Autodesk Inventor part; units mm, degrees
ref_plane "YZ Plane" through (0, 0, 0) normal (1, 0, 0) x (0, 1, 0)
ref_plane "XZ Plane" through (0, 0, 0) normal (0, 1, 0) x (-1, 0, 0)
ref_plane "XY Plane" through (0, 0, 0) normal (0, 0, 1) x (1, 0, 0)
sketch "Sketch1" plane through (0, 0, 0) normal (0, 0, 1) x (1, 0, 0)
  line L0 (0, 0) -> (115, 0)
  line L1 (115, 0) -> (115, 105)
  line L2 (115, 105) -> (0, 105)
  line L3 (0, 105) -> (0, 0)
  circle A0 centre (57.5, 52.5) radius 4.5
  line L4 (27.5, 22.5) -> (87.5, 22.5) construction
  line L5 (87.5, 22.5) -> (87.5, 82.5) construction
  line L6 (87.5, 82.5) -> (27.5, 82.5) construction
  line L7 (27.5, 82.5) -> (27.5, 22.5) construction
  circle A1 centre (87.5, 82.5) radius 2.5
  circle A2 centre (27.5, 82.5) radius 2.5
  circle A3 centre (27.5, 22.5) radius 2.5
  circle A4 centre (87.5, 22.5) radius 2.5
  point P0 (57.5, 0)
  point P1 (0, 52.5)
  point P2 (27.5, 52.5)
  point P3 (57.5, 82.5)
  dimension "d0" = 115
  dimension "d1" = 105
  dimension "d2" = 9
  dimension "d3" = 60
  dimension "d4" = 60
  dimension "d5" = 5
  dimension "d6" = 5
  dimension "d7" = 5
  dimension "d8" = 5
extrude "Extrusion1" add sketch "Sketch1" along normal blind 20
fillet "Fillet1" radius 20 4 edges at (0, 105, 10) (115, 105, 10) (115, 0, 10) (0, 0, 10)
sketch "Sketch5" plane through (0, 0, 20) normal (0, 0, 1) x (1, 0, 0)
  circle A0 centre (27.5, 82.5) radius 2.5
  circle A1 centre (87.5, 82.5) radius 2.5
  circle A2 centre (87.5, 22.5) radius 2.5
  circle A3 centre (27.5, 22.5) radius 2.5
  circle A4 centre (87.5, 82.5) radius 6.5
  circle A5 centre (87.5, 22.5) radius 6.5
  circle A6 centre (27.5, 22.5) radius 6.5
  circle A7 centre (27.5, 82.5) radius 6.5
  point P0 (0, 0)
  dimension "d18" = 13
  dimension "d19" = 13
  dimension "d20" = 13
  dimension "d21" = 13
extrude "Extrusion4" cut sketch "Sketch5" against normal blind 5 contours A0 | A1 | A2 | A3 | A4 | A5 | A6 | A7
properties part number "AA030" material "ABS Plastic"
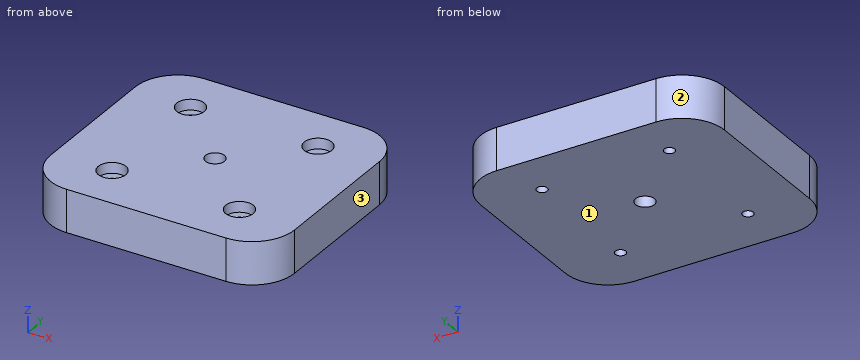
Check sheet for the modelled part. Datum: model origin and axes. Units: mm. Face numbers are marked on the shaded views. Give positions to 0.01 mm unless a question says otherwise; leave off trailing zeros. Write each loop counter-clockwise with the first axis right and the second up, starting at its lowest first coordinate (ties: lowest second). Pieces come first, ordered by that corner, then holes. Notation, with made-up numbers: (86, 1.25) -> (95, 1.25) arc R22 ccw to (95, 9.25) -> close; hole circle Ø1 at (-38, 55.25). An arc over 180 degrees is marked (long way). Write item = value, one per line.
Item 1: Sectioned sample at A-A on z = 17. Record the boundary of the cut face in (x, y).
Output:
outline = (0, 20) arc R20 ccw to (20, 0) -> (95, 0) arc R20 ccw to (115, 20) -> (115, 85) arc R20 ccw to (95, 105) -> (20, 105) arc R20 ccw to (0, 85) -> close; hole circle Ø13 at (27.5, 22.5); hole circle Ø13 at (27.5, 82.5); hole circle Ø9 at (57.5, 52.5); hole circle Ø13 at (87.5, 22.5); hole circle Ø13 at (87.5, 82.5)
Item 2: Scan lines: probe 1 along Y at (x, z) = (27.5, 5.75); probe 2 along X at (y, z) = (82.5, 10.75); probe 3 along Y at (x, z) = (24, 15.5). Record each from-to range of solid material in increasing order. Write a range as from..to.
Output:
probe_1 = 0..20, 25..80, 85..105
probe_2 = 0..25, 30..85, 90..115
probe_3 = 0..17.02, 27.98..77.02, 87.98..105
Item 3: Gauge pin test, flat ends, axial feed: pin 1 (3 mm diameter, centred on x = 27.5, y = 82.5, fed in from -Z); pin 2 (4 mm diameter, centred on x = 28, y = 83, fed in from +Z). Record the tip position at first contact, or that the pin passes through.
Output:
pin_1 = through
pin_2 = 15
Item 4: Release check for a two-part mould opening along X. For the marked faces 1, 2 and 3 record: +X half, -X half, draft (parallel to the pull), parting line (faces both ways), or undercut.
Output:
face_1 = draft
face_2 = -X half
face_3 = +X half
Item 5: Sectioned sample at D-D on y = 22.5. Record the boundary of the cut face in (x, z).
Output:
outline = (0, 0) -> (25, 0) -> (25, 15) -> (21, 15) -> (21, 20) -> (0, 20) -> close; (30, 0) -> (85, 0) -> (85, 15) -> (81, 15) -> (81, 20) -> (34, 20) -> (34, 15) -> (30, 15) -> close; (90, 0) -> (115, 0) -> (115, 20) -> (94, 20) -> (94, 15) -> (90, 15) -> close
Item 6: Sectioned sample at B-B on y = 52.5. Record the boundary of the cut face in (x, z).
Output:
outline = (0, 0) -> (53, 0) -> (53, 20) -> (0, 20) -> close; (62, 0) -> (115, 0) -> (115, 20) -> (62, 20) -> close
Item 7: Sectioned sample at C-C on x = 27.5. Record the boundary of the cut face in (y, z), and give its area (3 significant figures).
Output:
outline = (0, 0) -> (20, 0) -> (20, 15) -> (16, 15) -> (16, 20) -> (0, 20) -> close; (25, 0) -> (80, 0) -> (80, 15) -> (76, 15) -> (76, 20) -> (29, 20) -> (29, 15) -> (25, 15) -> close; (85, 0) -> (105, 0) -> (105, 20) -> (89, 20) -> (89, 15) -> (85, 15) -> close
area = 1,820 mm^2
